Geometry: final body of the model. Coordinates: model frame, mm. Face numbers are marked on the shaded views. A direction names the side the tool comes from. Give positions to 0.01 mm unless a question says otherwise; leave off trailing zeros. Order: outer loops, then holes, each group sorted by start corner. A loop starts at its lowest first (then second) coordinate and runs counter-clockwise, first axis right, second up. Notation, with made-up numbers: (68, 6) - (119, 6) arc R25 ccw to (119, 30) - close; hole circle Ø6 at (6, 71.25). An arc over 180 degrees is marked (long way). One line per item, written item: value.
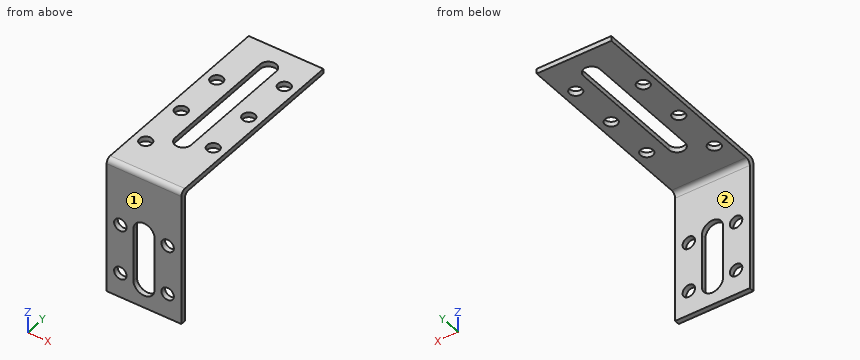
```python
from build123d import *

# Parameters (mm, degrees)
BOSS_EXTRU_1_DEPTH      = 15
CONG_1_R                = 2
ENL_V_MAT_EXTRU_1_REACH = 4
ESQUISSE2_R             = 2.5
ENL_V_MAT_EXTRU_2_REACH = 4
ESQUISSE4_R             = 2.5


with BuildPart() as part:
    # Esquisse1 → Boss.-Extru.1 (new body, symmetric)
    with BuildSketch(Plane(origin=(0, 0, 0), x_dir=(0, 0, -1), z_dir=(1, 0, 0))):
        Polygon((0, 0), (0, 80), (2, 80), (2, 2), (55, 2), (55, 0), align=None)
    extrude(amount=BOSS_EXTRU_1_DEPTH, both=True)

    # Congé1
    cong_1_edges = [part.edges().sort_by_distance(p)[0] for p in [
        (0, 0, 0),
        (0, 2, -2),
    ]]
    fillet(cong_1_edges, radius=CONG_1_R)

    # Esquisse2 → Enlèv. mat.-Extru.1 (cut, up to next)
    with BuildSketch(Plane(origin=(0, 2, 0), x_dir=(1, 0, 0), z_dir=(0, 1, 0)), mode=Mode.PRIVATE) as enl_v_mat_extru_1_sk1:
        with BuildLine():
            Line((4.25, 24.25), (4.25, 45.75))
            ThreePointArc((4.25, 45.75), (0, 50), (-4.25, 45.75))
            Line((-4.25, 45.75), (-4.25, 24.25))
            ThreePointArc((-4.25, 24.25), (0, 20), (4.25, 24.25))
        make_face()
    enl_v_mat_extru_1_tool1 = extrude(enl_v_mat_extru_1_sk1.sketch, amount=-ENL_V_MAT_EXTRU_1_REACH, mode=Mode.PRIVATE) & part.part
    add(enl_v_mat_extru_1_tool1.solids().sort_by_distance((0, 2, -35))[0], mode=Mode.SUBTRACT)
    # Esquisse2 → Enlèv. mat.-Extru.1 (cut, up to next)
    with BuildSketch(Plane(origin=(0, 2, 0), x_dir=(1, 0, 0), z_dir=(0, 1, 0)), mode=Mode.PRIVATE) as enl_v_mat_extru_1_sk2:
        with Locations((-9.5, 25)):
            Circle(ESQUISSE2_R)
    enl_v_mat_extru_1_tool2 = extrude(enl_v_mat_extru_1_sk2.sketch, amount=-ENL_V_MAT_EXTRU_1_REACH, mode=Mode.PRIVATE) & part.part
    add(enl_v_mat_extru_1_tool2.solids().sort_by_distance((-9.5, 2, -25))[0], mode=Mode.SUBTRACT)
    # Esquisse2 → Enlèv. mat.-Extru.1 (cut, up to next)
    with BuildSketch(Plane(origin=(0, 2, 0), x_dir=(1, 0, 0), z_dir=(0, 1, 0)), mode=Mode.PRIVATE) as enl_v_mat_extru_1_sk3:
        with Locations((-9.5, 45)):
            Circle(ESQUISSE2_R)
    enl_v_mat_extru_1_tool3 = extrude(enl_v_mat_extru_1_sk3.sketch, amount=-ENL_V_MAT_EXTRU_1_REACH, mode=Mode.PRIVATE) & part.part
    add(enl_v_mat_extru_1_tool3.solids().sort_by_distance((-9.5, 2, -45))[0], mode=Mode.SUBTRACT)
    # Esquisse2 → Enlèv. mat.-Extru.1 (cut, up to next)
    with BuildSketch(Plane(origin=(0, 2, 0), x_dir=(1, 0, 0), z_dir=(0, 1, 0)), mode=Mode.PRIVATE) as enl_v_mat_extru_1_sk4:
        with Locations((9.5, 45)):
            Circle(ESQUISSE2_R)
    enl_v_mat_extru_1_tool4 = extrude(enl_v_mat_extru_1_sk4.sketch, amount=-ENL_V_MAT_EXTRU_1_REACH, mode=Mode.PRIVATE) & part.part
    add(enl_v_mat_extru_1_tool4.solids().sort_by_distance((9.5, 2, -45))[0], mode=Mode.SUBTRACT)
    # Esquisse2 → Enlèv. mat.-Extru.1 (cut, up to next)
    with BuildSketch(Plane(origin=(0, 2, 0), x_dir=(1, 0, 0), z_dir=(0, 1, 0)), mode=Mode.PRIVATE) as enl_v_mat_extru_1_sk5:
        with Locations((9.5, 25)):
            Circle(ESQUISSE2_R)
    enl_v_mat_extru_1_tool5 = extrude(enl_v_mat_extru_1_sk5.sketch, amount=-ENL_V_MAT_EXTRU_1_REACH, mode=Mode.PRIVATE) & part.part
    add(enl_v_mat_extru_1_tool5.solids().sort_by_distance((9.5, 2, -25))[0], mode=Mode.SUBTRACT)

    # Esquisse4 → Enlèv. mat.-Extru.2 (cut, up to next)
    with BuildSketch(Plane(origin=(0, 0, -2), x_dir=(-1, 0, 0), z_dir=(0, 0, -1)), mode=Mode.PRIVATE) as enl_v_mat_extru_2_sk1:
        with Locations((-10, 65)):
            Circle(ESQUISSE4_R)
    enl_v_mat_extru_2_tool1 = extrude(enl_v_mat_extru_2_sk1.sketch, amount=-ENL_V_MAT_EXTRU_2_REACH, mode=Mode.PRIVATE) & part.part
    add(enl_v_mat_extru_2_tool1.solids().sort_by_distance((10, 65, -2))[0], mode=Mode.SUBTRACT)
    # Esquisse4 → Enlèv. mat.-Extru.2 (cut, up to next)
    with BuildSketch(Plane(origin=(0, 0, -2), x_dir=(-1, 0, 0), z_dir=(0, 0, -1)), mode=Mode.PRIVATE) as enl_v_mat_extru_2_sk2:
        with Locations((-10, 45)):
            Circle(ESQUISSE4_R)
    enl_v_mat_extru_2_tool2 = extrude(enl_v_mat_extru_2_sk2.sketch, amount=-ENL_V_MAT_EXTRU_2_REACH, mode=Mode.PRIVATE) & part.part
    add(enl_v_mat_extru_2_tool2.solids().sort_by_distance((10, 45, -2))[0], mode=Mode.SUBTRACT)
    # Esquisse4 → Enlèv. mat.-Extru.2 (cut, up to next)
    with BuildSketch(Plane(origin=(0, 0, -2), x_dir=(-1, 0, 0), z_dir=(0, 0, -1)), mode=Mode.PRIVATE) as enl_v_mat_extru_2_sk3:
        with Locations((-10, 25)):
            Circle(ESQUISSE4_R)
    enl_v_mat_extru_2_tool3 = extrude(enl_v_mat_extru_2_sk3.sketch, amount=-ENL_V_MAT_EXTRU_2_REACH, mode=Mode.PRIVATE) & part.part
    add(enl_v_mat_extru_2_tool3.solids().sort_by_distance((10, 25, -2))[0], mode=Mode.SUBTRACT)
    # Esquisse4 → Enlèv. mat.-Extru.2 (cut, up to next)
    with BuildSketch(Plane(origin=(0, 0, -2), x_dir=(-1, 0, 0), z_dir=(0, 0, -1)), mode=Mode.PRIVATE) as enl_v_mat_extru_2_sk4:
        with Locations((10, 55)):
            Circle(ESQUISSE4_R)
    enl_v_mat_extru_2_tool4 = extrude(enl_v_mat_extru_2_sk4.sketch, amount=-ENL_V_MAT_EXTRU_2_REACH, mode=Mode.PRIVATE) & part.part
    add(enl_v_mat_extru_2_tool4.solids().sort_by_distance((-10, 55, -2))[0], mode=Mode.SUBTRACT)
    # Esquisse4 → Enlèv. mat.-Extru.2 (cut, up to next)
    with BuildSketch(Plane(origin=(0, 0, -2), x_dir=(-1, 0, 0), z_dir=(0, 0, -1)), mode=Mode.PRIVATE) as enl_v_mat_extru_2_sk5:
        with Locations((10, 35)):
            Circle(ESQUISSE4_R)
    enl_v_mat_extru_2_tool5 = extrude(enl_v_mat_extru_2_sk5.sketch, amount=-ENL_V_MAT_EXTRU_2_REACH, mode=Mode.PRIVATE) & part.part
    add(enl_v_mat_extru_2_tool5.solids().sort_by_distance((-10, 35, -2))[0], mode=Mode.SUBTRACT)
    # Esquisse4 → Enlèv. mat.-Extru.2 (cut, up to next)
    with BuildSketch(Plane(origin=(0, 0, -2), x_dir=(-1, 0, 0), z_dir=(0, 0, -1)), mode=Mode.PRIVATE) as enl_v_mat_extru_2_sk6:
        with Locations((10, 15)):
            Circle(ESQUISSE4_R)
    enl_v_mat_extru_2_tool6 = extrude(enl_v_mat_extru_2_sk6.sketch, amount=-ENL_V_MAT_EXTRU_2_REACH, mode=Mode.PRIVATE) & part.part
    add(enl_v_mat_extru_2_tool6.solids().sort_by_distance((-10, 15, -2))[0], mode=Mode.SUBTRACT)
    # Esquisse4 → Enlèv. mat.-Extru.2 (cut, up to next)
    with BuildSketch(Plane(origin=(0, 0, -2), x_dir=(-1, 0, 0), z_dir=(0, 0, -1)), mode=Mode.PRIVATE) as enl_v_mat_extru_2_sk7:
        with BuildLine():
            Line((3.25, 70), (3.25, 22))
            ThreePointArc((3.25, 22), (0, 18.75), (-3.25, 22))
            Line((-3.25, 22), (-3.25, 70))
            ThreePointArc((-3.25, 70), (0, 73.25), (3.25, 70))
        make_face()
    enl_v_mat_extru_2_tool7 = extrude(enl_v_mat_extru_2_sk7.sketch, amount=-ENL_V_MAT_EXTRU_2_REACH, mode=Mode.PRIVATE) & part.part
    add(enl_v_mat_extru_2_tool7.solids().sort_by_distance((0, 46, -2))[0], mode=Mode.SUBTRACT)


solid = part.part
```
1) Material intervals for line 1 along X through (y, z) = (1.45, -25); line 2 along Z through (x, y) = (9.5, 0.85); line 3 along Z through (x, y) = (4, 24), sorted ascending.
Answers below:
line 1: -15 to -12, -7 to -4.25, 4.25 to 7, 12 to 15
line 2: -55 to -47.5, -42.5 to -27.5, -22.5 to -0.36
line 3: -2 to 0
2) Section B-B, the plane y = 15. Return loops of the section in (x, z).
Answers below:
outline: (-15, -2) - (-12.5, -2) - (-12.5, 0) - (-15, 0) - close; (-7.5, -2) - (15, -2) - (15, 0) - (-7.5, 0) - close
3) First-contact query: pin 1 (3 mm diameter, centred on x = -1, z = -40, fed in from -Y); pin 2 (4 mm diameter, centred on x = 3, y = 58.5, fed in from -Z); pin 3 (6.5 mm diameter, centred on x = 9.5, z = -25, fed in from +Y). Flat tips, straight axial feed; report the tip coordinate or a pass-through.
Answers below:
pin 1: through
pin 2: z = -2
pin 3: y = 2
4) Set-up query: the marked faces 1 and 2. Return all of +Z, -Z, +X, -X, +Y, -Y with unobstructed straight access to the full face (end or side cutting, diameter ignored); none if empty.
Answers below:
face 1: +Z, -Z, +X, -X, -Y
face 2: -Z, +X, -X, +Y
5) Section C-C, the plane x = 9.5. Return loops of the section in (y, z).
Answers below:
outline: (0, -55) - (2, -55) - (2, -47.5) - (0, -47.5) - close; (0, -42.5) - (2, -42.5) - (2, -27.5) - (0, -27.5) - close; (0, -22.5) - (2, -22.5) - (2, -4) arc R2 cw to (4, -2) - (22.55, -2) - (22.55, 0) - (2, 0) arc R2 ccw to (0, -2) - close; (27.45, -2) - (42.55, -2) - (42.55, 0) - (27.45, 0) - close; (47.45, -2) - (62.55, -2) - (62.55, 0) - (47.45, 0) - close; (67.45, -2) - (80, -2) - (80, 0) - (67.45, 0) - close
6) Section D-D, the plane y = 55. Return loops of the section in (x, z).
Answers below:
outline: (-15, -2) - (-12.5, -2) - (-12.5, 0) - (-15, 0) - close; (-7.5, -2) - (-3.25, -2) - (-3.25, 0) - (-7.5, 0) - close; (3.25, -2) - (15, -2) - (15, 0) - (3.25, 0) - close
7) Section A-A, the plane z = -36. Return loops of the section in (x, y), then the cut area to 3 significant figures.
Answers below:
outline: (-15, 0) - (-4.25, 0) - (-4.25, 2) - (-15, 2) - close; (4.25, 0) - (15, 0) - (15, 2) - (4.25, 2) - close
area: 43.0 mm^2
